```python
from build123d import *

# Parameters (mm, degrees)
SKETCH2_R           = 50
BOSS_EXTRUDE1_DEPTH = 10
BOSS_EXTRUDE2_DEPTH = 10
CIRPATTERN1_COUNT   = 6


with BuildPart() as part:
    # Sketch2 → Boss-Extrude1 (new body)
    with BuildSketch(Plane.XY):
        Circle(SKETCH2_R)
    extrude(amount=-BOSS_EXTRUDE1_DEPTH)

    # Sketch3 → Boss-Extrude2 (add)
    with BuildSketch(Plane.XY):
        Polygon((-22.5, 262.5), (-22.5, 0), (0, 0), (22.5, 0), (22.5, 262.5), (65.801270189, 287.5), (55.801270189, 304.820508076), (22.5, 285.594010768), (22.5, 312.5), (-22.5, 312.5), (-22.5, 285.594010768), (-55.801270189, 304.820508076), (-65.801270189, 287.5), align=None)
    boss_extrude2 = extrude(amount=-BOSS_EXTRUDE2_DEPTH)

    # CirPattern1: Boss-Extrude2 ×6 about axis
    cirpattern1_axis = Axis((0, 0, 0), (0, 0, 1))
    for i in range(1, CIRPATTERN1_COUNT):
        add(boss_extrude2.rotate(cirpattern1_axis, i * 360 / CIRPATTERN1_COUNT))


solid = part.part
```
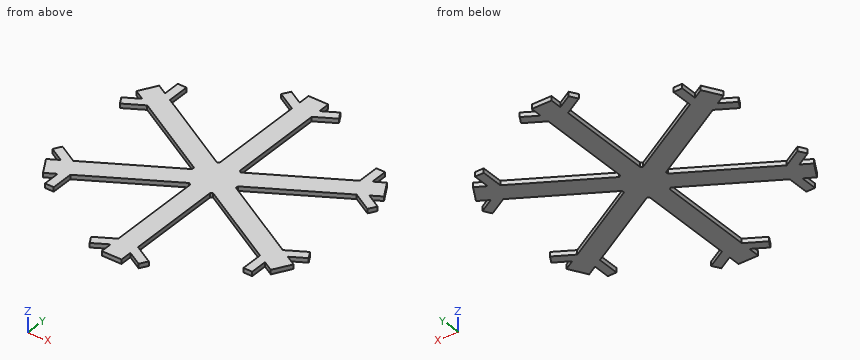
Geometry: final body of the model. Coordinates: model frame, mm. Round coordinates to 2 decimals unless told otherwise and drop trailing zeros. Write each loop counter-clockwise with the first axis right and the second up, starting at its lowest first coordinate (ties: lowest second). Pieces come first, ordered by that corner, then holes.
Item 1: Section query C-C (y = -224). Return loops of the section in (x, z), plus the area to 3 significant figures.
Item 2: Pin query (flat end, axial travel): P1, Ø3, axis at x = -230.5, z = -2.5, coming from the +Y side; P2, Ø5, axis at y = 181.5, z = -4, coming from the +X side; P3, Ø5, axis at x = 85.5, z = -5, coming from the -Y side. Return the tip coordinate at first contact, or that it passes through.
Item 3: Section query A-A (x = 92.5). Return loops of the section in (y, z), plus the area to 3 significant figures.
Item 4: Section query B-B (y = -58.5). Return loops of the section in (x, z), plus the area to 3 significant figures.
Item 5: Material intervals for L1, parallel to X at y = -184.5, z = -8.5; L2, parallel to X at y = -127.5, z = -1; L3, parallel to Y at x = 261.5, z = -6, sorted ascending.
Completed:
1. outline: (-22.5, -10) - (22.5, -10) - (22.5, 0) - (-22.5, 0) - close
1. area: 450 mm2
2. P1: stops at y = 200.74
2. P2: stops at x = 236.08
2. P3: stops at y = -76.79
3. outline: (-79.39, -10) - (-27.42, -10) - (-27.42, 0) - (-79.39, 0) - close; (27.42, -10) - (79.39, -10) - (79.39, 0) - (27.42, 0) - close
3. area: 1,040 mm2
4. outline: (-146.32, -10) - (-56.32, -10) - (-56.32, 0) - (-146.32, 0) - close; (-22.5, -10) - (22.5, -10) - (22.5, 0) - (-22.5, 0) - close; (56.32, -10) - (146.32, -10) - (146.32, 0) - (56.32, 0) - close
4. area: 2,250 mm2
5. L1: x = -236.08 to -216.08, -22.5 to 22.5, 216.08 to 236.08
5. L2: x = -265.84 to -175.84, -22.5 to 22.5, 175.84 to 265.84
5. L3: y = -172.07 to -125, -121.63 to -98.53, 98.53 to 121.63, 125 to 172.07
